Input: part model. Units: mm. Frame: model coordinates. A direction names the side the tool comes from. Give positions to 0.01 mm unless a question says otherwise; leave off trailing zeros. Loops run counter-clockwise (first coordinate to the right, second up) from the corner with the lowest first, then second, coordinate; pieces in that order, holes last. Notation, with made-up numbers: (67.25, 69.5) - (92.25, 69.5) arc R16 cw to (92.25, 99.5) - close; hole circle Ø4 at (-31.5, -2.5). An arc over 180 degrees is marked (long way). One line per item, written item: value.
from build123d import *

# Parameters (mm, degrees)
SKETCH1_W           = 245
SKETCH1_H           = 180.5
BOSS_EXTRUDE1_DEPTH = 10
SKETCH1_5_R         = 1.7
CUT_EXTRUDE2_DEPTH  = 153.483810616
SKETCH2_W           = 120
SKETCH2_H           = 6
BOSS_EXTRUDE3_DEPTH = 30
SKETCH3_W           = 120
SKETCH3_H           = 9
BOSS_EXTRUDE4_DEPTH = 20
SKETCH4_R           = 2
CUT_EXTRUDE4_DEPTH  = 156.084855805
SKETCH7_R           = 3.25
CUT_EXTRUDE5_DEPTH  = 156.084855805
SKETCH9_R           = 1.7
CUT_EXTRUDE6_DEPTH  = 158.325498569
SKETCH10_R          = 2
CUT_EXTRUDE7_DEPTH  = 158.325498569


with BuildPart() as part:
    # Sketch1 → Boss-Extrude1 (new body)
    with BuildSketch(Plane(origin=(0, 0, 0), x_dir=(1, 0, 0), z_dir=(0, 1, 0))):
        Rectangle(SKETCH1_W, SKETCH1_H)
    extrude(amount=-BOSS_EXTRUDE1_DEPTH)

    # Sketch1_5 → Cut-Extrude2 (cut, through all)
    with BuildSketch(Plane(origin=(0, 0, 0), x_dir=(1, 0, 0), z_dir=(0, 1, 0))):
        with Locations(Location((-88.5, -67.75, 0), (0, 0, 270))):
            Circle(SKETCH1_5_R)
        with Locations(Location((-45, -67.75, 0), (0, 0, 270))):
            Circle(SKETCH1_5_R)
        with Locations(Location((-8.5, -67.75, 0), (0, 0, 270))):
            Circle(SKETCH1_5_R)
        with Locations(Location((35, -67.75, 0), (0, 0, 270))):
            Circle(SKETCH1_5_R)
        with Locations(Location((71.5, -67.75, 0), (0, 0, 270))):
            Circle(SKETCH1_5_R)
        with Locations(Location((115, 67.75, 0), (0, 0, 270))):
            Circle(SKETCH1_5_R)
        with Locations(Location((71.5, 67.75, 0), (0, 0, 270))):
            Circle(SKETCH1_5_R)
        with Locations(Location((-8.5, 67.75, 0), (0, 0, 270))):
            Circle(SKETCH1_5_R)
        with Locations(Location((-45, 67.75, 0), (0, 0, 270))):
            Circle(SKETCH1_5_R)
        with Locations(Location((-88.5, 67.75, 0), (0, 0, 270))):
            Circle(SKETCH1_5_R)
        with Locations(Location((115, -67.75, 0), (0, 0, 270))):
            Circle(SKETCH1_5_R)
        with Locations(Location((35, 67.75, 0), (0, 0, 270))):
            Circle(SKETCH1_5_R)
    extrude(amount=-CUT_EXTRUDE2_DEPTH, mode=Mode.SUBTRACT)

    # Sketch2 → Boss-Extrude3 (add)
    with BuildSketch(Plane.XZ.offset(10)):
        with Locations((-33.5, 0)):
            Rectangle(SKETCH2_W, SKETCH2_H)
    extrude(amount=BOSS_EXTRUDE3_DEPTH)

    # Sketch3 → Boss-Extrude4 (add)
    with BuildSketch(Plane.XZ.offset(10)):
        with Locations((-33.5, 0)):
            Rectangle(SKETCH3_W, SKETCH3_H)
    extrude(amount=BOSS_EXTRUDE4_DEPTH)

    # Sketch4 → Cut-Extrude4 (cut, through all)
    with BuildSketch(Plane.XZ.offset(10)):
        with Locations(Location((-86, 15, 0), (0, 0, 270))):
            Circle(SKETCH4_R)
        with Locations(Location((19, 15, 0), (0, 0, 270))):
            Circle(SKETCH4_R)
        with Locations(Location((19, -15, 0), (0, 0, 270))):
            Circle(SKETCH4_R)
        with Locations(Location((-86, -15, 0), (0, 0, 270))):
            Circle(SKETCH4_R)
    extrude(amount=-CUT_EXTRUDE4_DEPTH, mode=Mode.SUBTRACT)

    # Sketch7 → Cut-Extrude5 (cut, through all)
    with BuildSketch(Plane.XZ.offset(10)):
        with Locations(Location((-109.8, 77.55, 0), (0, 0, 270))):
            Circle(SKETCH7_R)
        with Locations(Location((0, 77.55, 0), (0, 0, 270))):
            Circle(SKETCH7_R)
        with Locations(Location((109.8, 77.55, 0), (0, 0, 270))):
            Circle(SKETCH7_R)
        with Locations(Location((-109.8, -77.55, 0), (0, 0, 90))):
            Circle(SKETCH7_R)
        with Locations(Location((0, -77.55, 0), (0, 0, 90))):
            Circle(SKETCH7_R)
        with Locations(Location((109.8, -77.55, 0), (0, 0, 90))):
            Circle(SKETCH7_R)
    extrude(amount=-CUT_EXTRUDE5_DEPTH, mode=Mode.SUBTRACT)

    # Sketch9 → Cut-Extrude6 (cut, through all)
    with BuildSketch(Plane(origin=(0, 0, 0), x_dir=(1, 0, 0), z_dir=(0, 1, 0))):
        with Locations(Location((41.5, 20, 0), (0, 0, 270))):
            Circle(SKETCH9_R)
        with Locations(Location((63.5, -20, 0), (0, 0, 270))):
            Circle(SKETCH9_R)
        with Locations(Location((-38.5, 20, 0), (0, 0, 270))):
            Circle(SKETCH9_R)
        with Locations(Location((-16.5, -20, 0), (0, 0, 270))):
            Circle(SKETCH9_R)
        with Locations(Location((-118.5, 20, 0), (0, 0, 270))):
            Circle(SKETCH9_R)
        with Locations(Location((-96.5, -20, 0), (0, 0, 270))):
            Circle(SKETCH9_R)
        with BuildLine():
            Line((58.25, 59.85), (58.25, 44.85))
            ThreePointArc((58.25, 44.85), (53.25, 39.85), (48.25, 44.85))
            Line((48.25, 44.85), (48.25, 59.85))
            ThreePointArc((48.25, 59.85), (53.25, 64.85), (58.25, 59.85))
        make_face()
        with BuildLine():
            Line((-21.75, 59.85), (-21.75, 44.85))
            ThreePointArc((-21.75, 44.85), (-26.75, 39.85), (-31.75, 44.85))
            Line((-31.75, 44.85), (-31.75, 59.85))
            ThreePointArc((-31.75, 59.85), (-26.75, 64.85), (-21.75, 59.85))
        make_face()
        with BuildLine():
            Line((-101.75, 59.85), (-101.75, 44.85))
            ThreePointArc((-101.75, 44.85), (-106.75, 39.85), (-111.75, 44.85))
            Line((-111.75, 44.85), (-111.75, 59.85))
            ThreePointArc((-111.75, 59.85), (-106.75, 64.85), (-101.75, 59.85))
        make_face()
    extrude(amount=-CUT_EXTRUDE6_DEPTH, mode=Mode.SUBTRACT)

    # Sketch10 → Cut-Extrude7 (cut, through all)
    with BuildSketch(Plane(origin=(0, 0, 0), x_dir=(1, 0, 0), z_dir=(0, 1, 0))):
        with Locations(Location((85.5, -33, 0), (0, 0, 270))):
            Circle(SKETCH10_R)
        with Locations(Location((85.5, 33, 0), (0, 0, 270))):
            Circle(SKETCH10_R)
    extrude(amount=-CUT_EXTRUDE7_DEPTH, mode=Mode.SUBTRACT)


solid = part.part
Item 1: Draft query along Z for faces 4 (the face through (-112.54, -5.07, -75.8)), 5 (the face through (-34, -40, 0)), 6 (the face through (-34, -20, 4.5)). Return one class per face: pulls with the +Z half, pulls with the -Z half, needs draft (parallel to the pull), parting line crosses it, or undercut.
Verdict:
face 4: undercut
face 5: needs draft
face 6: pulls with the +Z half
Item 2: Section D-D, the plane x = -78. Output: boundary loops of the cut face in (y, z).
Verdict:
outline: (-40, -3) - (-30, -3) - (-30, -4.5) - (-10, -4.5) - (-10, -90.25) - (0, -90.25) - (0, 90.25) - (-10, 90.25) - (-10, 4.5) - (-30, 4.5) - (-30, 3) - (-40, 3) - close
Item 3: Section A-A, the plane x = 0. Output: boundary loops of the cut face in (y, z).
Verdict:
outline: (-40, -3) - (-30, -3) - (-30, -4.5) - (-10, -4.5) - (-10, -74.3) - (0, -74.3) - (0, 74.3) - (-10, 74.3) - (-10, 4.5) - (-30, 4.5) - (-30, 3) - (-40, 3) - close; (-10, -90.25) - (0, -90.25) - (0, -80.8) - (-10, -80.8) - close; (-10, 80.8) - (0, 80.8) - (0, 90.25) - (-10, 90.25) - close
Item 4: Material intervals for L1, parallel to X at y = -5, z = -77; L2, parallel to X at y = -3, z = 20; L3, parallel to Z at x = 71.5, y = -7, sorted ascending.
Verdict:
L1: x = -122.5 to -113, -106.6 to -3.2, 3.2 to 106.6, 113 to 122.5
L2: x = -122.5 to -98.2, -94.8 to -18.2, -14.8 to 61.8, 65.2 to 122.5
L3: z = -90.25 to -69.45, -66.05 to 66.05, 69.45 to 90.25
Item 5: Section B-B, the plane z = -53.5. Output: boundary loops of the cut face in (x, y).
Verdict:
outline: (-122.5, -10) - (-111.75, -10) - (-111.75, 0) - (-122.5, 0) - close; (-101.75, -10) - (-31.75, -10) - (-31.75, 0) - (-101.75, 0) - close; (-21.75, -10) - (48.25, -10) - (48.25, 0) - (-21.75, 0) - close; (58.25, -10) - (122.5, -10) - (122.5, 0) - (58.25, 0) - close
Item 6: Access query for faces 1 (the face through (-26.64, -4.93, -39.85)), 2 (the face through (-34, -35, 3)), 3 (the face through (-34, -35, -3)). Directions: +Z, -Z, +X, -X, +Y, -Y. A direction counts if a zero-diameter tool reaches every point of the face in a straight line with its end or side. Return the directions, or none.
Verdict:
face 1: +Y, -Y
face 2: +Z, +X, -X, -Y
face 3: -Z, +X, -X, -Y
Item 7: Pin query (flat end, axial travel): P1, Ø4.5, axis at y = -21, z = 2, coming from the +X side; P2, Ø5.5, axis at x = 63.5, z = 20, coming from the +Y side; P3, Ø4.5, axis at x = -38.5, z = -20, coming from the -Y side; P4, Ø10, axis at y = -32, z = -1, coming from the -X side. Return the tip coordinate at first contact, or that it passes through.
Verdict:
P1: stops at x = 26.5
P2: stops at y = 0
P3: stops at y = -10
P4: stops at x = -93.5
Item 8: Section C-C, the plane y = -5. Count the separate pieces of the cut face and the enclosed holes in it, and give its area (3 significant figures).
Verdict:
separate pieces: 1
enclosed holes: 33
area: 43,100 mm^2
